For this review, take the finished solid that the model builds, in its own axes (mm). Face numbers are marked on the shaded views. A direction names the side the tool comes from. Give positions to 0.01 mm unless a question says otherwise; leave off trailing zeros. Loops run counter-clockwise (first coordinate to the right, second up) from the corner with the lowest first, then second, coordinate; pieces in that order, holes last. Notation, with made-up numbers: M 66.5,5 L 89.5,5 A20 ccw 89.5,26 Z; hole C 9,-29.5 d11. An arc over 180 degrees is marked long. Use CSV: the item, a comma, the result in double quotes. Start each with the question number.
1. Take a section at A-A, the plane y = 7. Write out the cut boundary in (x, z), and give its area (3 significant figures).
2. The part is to be moulded in two halves that separate along X. For the marked faces 1, 2, 3 and 4, say which applies: pulls with the +X half, pulls with the -X half, needs draft (parallel to the pull), parting line crosses it, or undercut.
3. Insertion check: P1, Ø4, axis at y = 4, z = 0.5, coming from the +X side; P2, Ø4, axis at x = 6.5, y = 7.5, coming from the +Z side. Each pin has a flat end and moves straight along its axis. Give the tip position at first contact, or say it passes through.
4. Take a section at C-C, the plane y = 3. Write out the cut boundary in (x, z), and give its area (3 significant figures).
5. Take a section at B-B, the plane x = 7. Write out the cut boundary in (y, z).
6. Take a section at D-D, the plane z = -11. Write out the cut boundary in (x, y).
7. To check wall thickness, follow line 1 (Z direction, x = 4.5, y = 10.25); line 2 (X direction, y = 9, z = 9); line 3 (X direction, y = 7, z = -11.1). State the ranges of each line that lie inside material, in increasing order. Write a range as [from, to].
8. Tool access review of the marked faces 5 and 6: name each direction out of +Z, -Z, +X, -X, +Y, -Y from which nothing blocks a thin tool from reaching the whole face with its end or side.
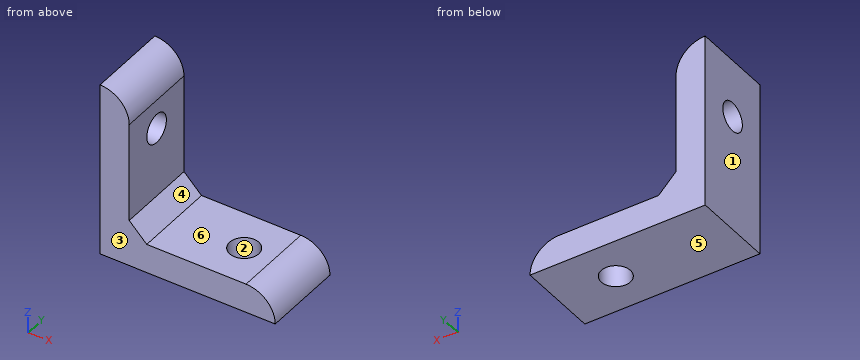
from build123d import *

# Parameters (mm, degrees)
F1_DEPTH = 14
F2_R     = 2.5
F3_DEPTH = 5
F4_R     = 2.5
F5_DEPTH = 5


with BuildPart() as f1:
    # F0 (on Front) → F1 (new body)
    with BuildSketch(Plane.XZ):
        Polygon((-6.288725, 7.019924), (-11.288725, 7.019924), (-11.288725, -12.980076), (8.711275, -12.980076), (8.711275, -7.980076), (-3.288725, -7.980076), (-6.288725, -4.980076), align=None)
        with BuildLine():
            Line((8.711275, -7.980076), (8.711275, -12.980076))
            Line((8.711275, -12.980076), (18.711275, -12.980076))
            ThreePointArc((18.711275, -12.980076), (17.246809, -9.444542), (13.711275, -7.980076))
            Line((13.711275, -7.980076), (8.711275, -7.980076))
        make_face()
        with BuildLine():
            ThreePointArc((-6.288725, 12.019924), (-7.753191, 15.555458), (-11.288725, 17.019924))
            Line((-11.288725, 17.019924), (-11.288725, 7.019924))
            Line((-11.288725, 7.019924), (-6.288725, 7.019924))
            Line((-6.288725, 7.019924), (-6.288725, 12.019924))
        make_face()
    extrude(amount=-F1_DEPTH)

    # F2 (on face) → F3 (cut)
    with BuildSketch(Plane(origin=(-11.288725, 0, 0), x_dir=(0, -1, 0), z_dir=(-1, 0, 0))):
        with Locations((-7, 7.019924)):
            Circle(F2_R)
    extrude(amount=-F3_DEPTH, mode=Mode.SUBTRACT)

    # F4 (on face) → F5 (cut)
    with BuildSketch(Plane(origin=(0, 0, -12.980076), x_dir=(1, 0, 0), z_dir=(0, 0, -1))):
        with Locations((8.711275, -7)):
            Circle(F4_R)
    extrude(amount=-F5_DEPTH, mode=Mode.SUBTRACT)


solid = f1.part
Result set:
1,outline,"M -11.29,-12.98 L 6.21,-12.98 L 6.21,-7.98 L -3.29,-7.98 L -6.29,-4.98 L -6.29,4.52 L -11.29,4.52 Z; M -11.29,9.52 L -6.29,9.52 L -6.29,12.02 A5 ccw -11.29,17.02 Z; M 11.21,-12.98 L 18.71,-12.98 A5 ccw 13.71,-7.98 L 11.21,-7.98 Z"
1,area,"219 mm2"
2,face 1,"pulls with the -X half"
2,face 2,"undercut"
2,face 3,"needs draft"
2,face 4,"pulls with the +X half"
3,P1,"x = -6.29"
3,P2,"z = -7.98"
4,outline,"M -11.29,-12.98 L 18.71,-12.98 A5 ccw 13.71,-7.98 L -3.29,-7.98 L -6.29,-4.98 L -6.29,12.02 A5 ccw -11.29,17.02 Z"
4,area,"269 mm2"
5,outline,"M 0,-12.98 L 5.18,-12.98 L 5.18,-7.98 L 0,-7.98 Z; M 8.82,-12.98 L 14,-12.98 L 14,-7.98 L 8.82,-7.98 Z"
6,outline,"M -11.29,0 L 18.3,0 L 18.3,14 L -11.29,14 Z; hole C 8.71,7 d5"
7,line 1,"[-12.98, -7.98]"
7,line 2,"[-11.29, -6.29]"
7,line 3,"[-11.29, 6.21], [11.21, 18.34]"
8,face 5,"-Z, +X, -X, +Y, -Y"
8,face 6,"+Z, +X, +Y, -Y"
